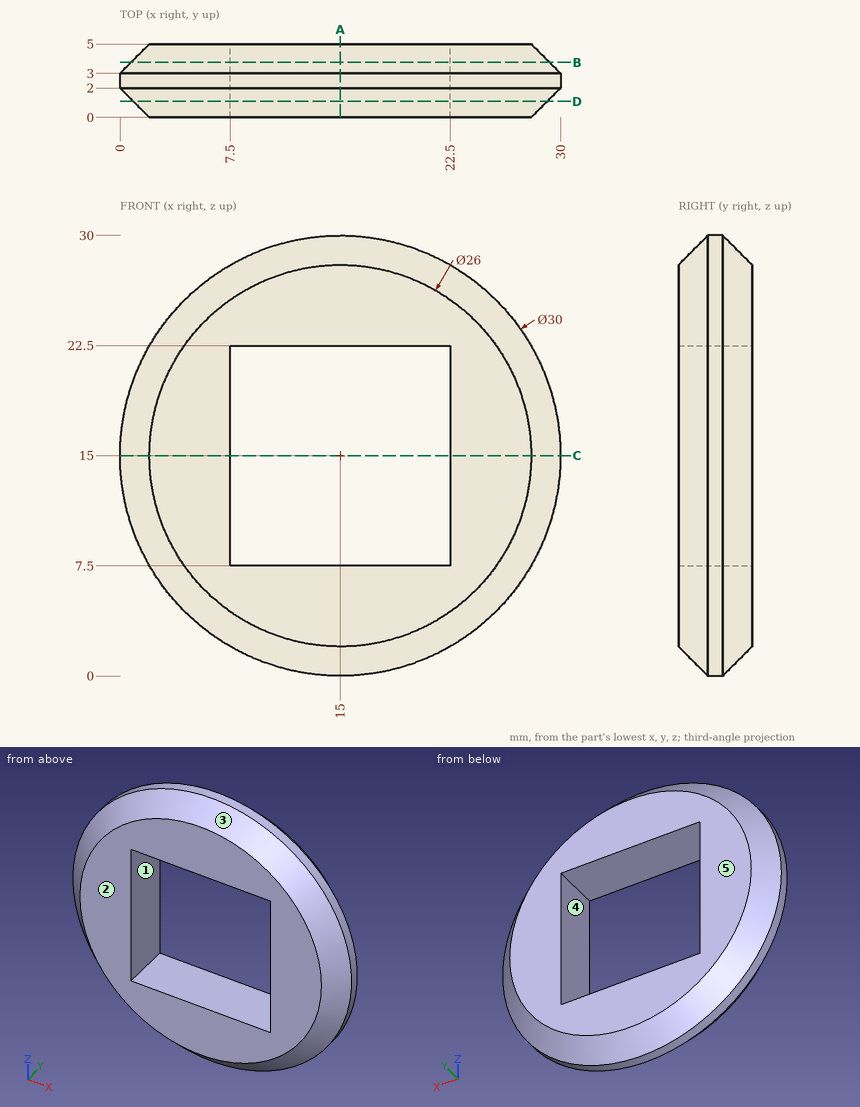
Job drawing, mm, ordinate dimensions from the low corner. One solid piece. A direction names the side the tool comes from. Give positions to 0.01 mm unless a question says otherwise; leave off trailing zeros. Loops run counter-clockwise (first coordinate to the right, second up) from the corner with the lowest first, then second, coordinate; pieces in that order, holes last. Notation, with made-up numbers: (31.25, 9.5) -> (82.25, 9.5) arc R35 ccw to (82.25, 44.5) -> close; hole circle Ø7 at (-26.5, 64.25). An arc over 180 degrees is marked (long way). Write each question's results on one line, items separated by ' | '.
(1) Flat gauge pins, fed straight in: pin 1 Ø1.5 at (x, z) = (5.5, 4.5) entering from -Y; pin 2 Ø1.5 at (x, y) = (18.5, 3) entering from +Z; pin 3 Ø1.5 at (x, y) = (17.5, 3.5) entering from +Z. Where does each tip first touch, or does it go through?
Geometry results:
pin 1: stops at y = 0.41 | pin 2: stops at z = 29.75 | pin 3: stops at z = 29.87
(2) Cut at C-C on z = 15. List the corners of the cut face in (x, y).
Geometry results:
outline: (0, 2) -> (2, 0) -> (7.5, 0) -> (7.5, 5) -> (2, 5) -> (0, 3) -> close; (22.5, 0) -> (28, 0) -> (30, 2) -> (30, 3) -> (28, 5) -> (22.5, 5) -> close
(3) Cut at D-D on y = 1.1. List the corners of the cut face in (x, z), and give its area (3 significant figures).
Geometry results:
outline: circle Ø28.2 at (15, 15); hole (7.5, 7.5) -> (22.5, 7.5) -> (22.5, 22.5) -> (7.5, 22.5) -> close | area: 400 mm²
(4) Tool access for the marked faces 4 and 5: list every direction of +Z, -Z, +X, -X, +Y, -Y with a clear straight run to the whole face (end or side of a thin tool).
Geometry results:
face 4: +Y, -Y | face 5: +Z, -Z, +X, -X, +Y
(5) Cut at B-B on y = 3.75. List the corners of the cut face in (x, z), and give its area (3 significant figures).
Geometry results:
outline: circle Ø28.5 at (15, 15); hole (7.5, 7.5) -> (22.5, 7.5) -> (22.5, 22.5) -> (7.5, 22.5) -> close | area: 413 mm²
(6) Probe line 1 along Z through (x, y) = (15.25, 2.35); line 2 along X through (y, z) = (2.55, 14.5); line 3 along Z through (x, y) = (19.25, 4.75). List the from-to ranges inside material, lowest first.
Geometry results:
line 1: z = 0 to 7.5, 22.5 to 30 | line 2: x = 0.01 to 7.5, 22.5 to 29.99 | line 3: z = 2.45 to 7.5, 22.5 to 27.55
(7) Pull direction Z, two halves, no side cores. Call the marked faces 1, 2 and 3: released by +Z, released by -Z, zero draft, split by the parting line, or undercut.
Geometry results:
face 1: undercut | face 2: zero draft | face 3: split by the parting line
(8) Cut at A-A on x = 15. List the corners of the cut face in (y, z).
Geometry results:
outline: (0, 2) -> (2, 0) -> (3, 0) -> (5, 2) -> (5, 7.5) -> (0, 7.5) -> close; (0, 22.5) -> (5, 22.5) -> (5, 28) -> (3, 30) -> (2, 30) -> (0, 28) -> close
